Can you work these out from the model? Positions are in its coordinate system, mm. Face numbers are marked on the shaded views. A direction names the side the tool comes from. Give positions to 0.01 mm unless a question says otherwise; leave off trailing zeros. Order: outer loops, then holes, each group sorted by start corner. A loop starts at its lowest first (then second) coordinate and runs counter-clockwise, first axis right, second up. Notation, with made-up numbers: (55, 4.25) - (92, 4.25) arc R13 ccw to (92, 17.25) - close; hole circle Ø7 at (33, -28.75). An arc over 180 degrees is marked (long way). Use one line per item in the form item = value. Start each with the question number.
1) Suppose I cut it at B-B, the plane z = 4.5. Write out the boundary of the cut face in (x, y).
2) Which directions (+Z, -Z, +X, -X, +Y, -Y) give clear straight access to the entire face, cutting with the end or side of a thin tool? Please do the marked faces 3, 4 and 5.
3) Suppose I cut it at C-C, the plane z = -83.5. State how many separate pieces and enclosed holes the cut face has, and give its area (3 significant figures).
4) Please list where these lines run through material, in increasing order: probe 1 along X at (y, z) = (9.65, -70); probe 2 along X at (y, z) = (21, -66); probe 3 along X at (y, z) = (7, -24).
5) For pin 1 (0.6 mm diameter, centred on x = 0, y = 19.5, fed in from -Z); pin 2 (1.1 mm diameter, centred on x = -38, y = 20.5, fed in from +Z); pin 3 (3.5 mm diameter, centred on x = -39, z = -70.5, fed in from -Y), each with a flat end and sliding along its axis, tell me the tip position at first contact or that it passes through.
6) Suppose I cut it at A-A, the plane x = 21. Write out the boundary of the cut face in (y, z).
7) We'd pull the mould along X, two halves only. Please class the marked faces 1 and 2: released by +X, released by -X, zero draft, split by the parting line, or undercut.
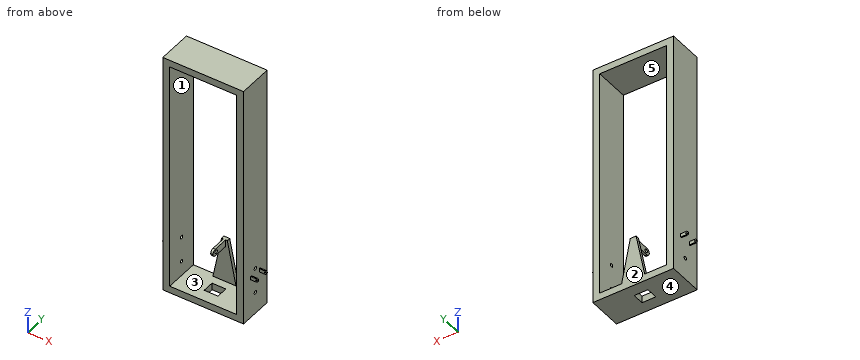
```python
from build123d import *

# Parameters (mm, degrees)
SKETCH1_W            = 70
SKETCH1_H            = 212
SKETCH1_W_2          = 58
SKETCH1_H_2          = 200
BOSS_EXTRUDE1_DEPTH  = 30
SKETCH10_W           = 2
SKETCH10_H           = 6
BOSS_EXTRUDE3_DEPTH  = 16
FILLET2_R            = 3
SKETCH2_R            = 1.5
CUT_EXTRUDE1_DEPTH   = 131.52202895
CUT_EXTRUDE2_REACH   = 218.954
SKETCH3_W            = 12
SKETCH3_H            = 10
SKETCH11_W           = 3
SKETCH11_H           = 1
BOSS_EXTRUDE4_DEPTH  = 6.3
FILLET3_R            = 1.5
SKETCH12_R           = 0.5
CUT_EXTRUDE3_DEPTH   = 116.683577146
FILLET3_OF_MIRROR1_R = 1.5


with BuildPart() as part:
    # Sketch1 → Boss-Extrude1 (new body)
    with BuildSketch(Plane(origin=(0, 0, 0), x_dir=(1, 0, 0), z_dir=(0, 1, 0))):
        Rectangle(SKETCH1_W, SKETCH1_H)
        Rectangle(SKETCH1_W_2, SKETCH1_H_2, mode=Mode.SUBTRACT)
    extrude(amount=BOSS_EXTRUDE1_DEPTH)

    # Sketch7 → Loft3 section 0
    with BuildSketch(Plane.XY.offset(-100)):
        with BuildLine():
            Line((-10, 30), (10, 30))
            Line((10, 30), (10, 27))
            Line((10, 27), (-10, 27))
            Line((-10, 27), (-10, 30))
        make_face()
    # Sketch8 → Loft3 section 1
    with BuildSketch(Plane.XY.offset(-62)):
        with BuildLine():
            Line((-2.5, 30), (2.5, 30))
            Line((2.5, 30), (2.5, 27))
            Line((2.5, 27), (-2.5, 27))
            Line((-2.5, 27), (-2.5, 30))
        make_face()
    loft()

    # Sketch10 → Boss-Extrude3 (add)
    with BuildSketch(Plane.XZ.offset(-27)):
        with Locations((0, -65)):
            Rectangle(SKETCH10_W, SKETCH10_H)
    extrude(amount=BOSS_EXTRUDE3_DEPTH)

    # Fillet2
    fillet2_edges = [part.edges().sort_by_distance(p)[0] for p in [
        (0, 11, -68),
        (0, 11, -62),
    ]]
    fillet(fillet2_edges, radius=FILLET2_R - 0.0001)  # a hair under: the kernel refuses the full size

    # Sketch2 → Cut-Extrude1 (cut, through all)
    with BuildSketch(Plane(origin=(35, 0, 0), x_dir=(0, 0, -1), z_dir=(1, 0, 0))):
        with Locations(Location((65, 15, 0), (0, 0, 270))):
            Circle(SKETCH2_R)
        with Locations((87, 15)):
            Circle(SKETCH2_R)
    extrude(amount=-CUT_EXTRUDE1_DEPTH, mode=Mode.SUBTRACT)

    # Sketch3 → Cut-Extrude2 (cut, up to next)
    with BuildSketch(Plane(origin=(0, 0, -106), x_dir=(-1, 0, 0), z_dir=(0, 0, -1)), mode=Mode.PRIVATE) as cut_extrude2_sk1:
        with Locations((0, 15)):
            Rectangle(SKETCH3_W, SKETCH3_H)
    cut_extrude2_tool1 = extrude(cut_extrude2_sk1.sketch, amount=-CUT_EXTRUDE2_REACH, mode=Mode.PRIVATE) & part.part
    add(cut_extrude2_tool1.solids().sort_by_distance((0, 15, -106))[0], mode=Mode.SUBTRACT)

    # Sketch11 → Boss-Extrude4 (add)
    with BuildSketch(Plane(origin=(35, 0, 0), x_dir=(0, 0, -1), z_dir=(1, 0, 0))):
        with Locations((70, 20.5)):
            Rectangle(SKETCH11_W, SKETCH11_H)
        with Locations((70, 9.5)):
            Rectangle(SKETCH11_W, SKETCH11_H)
    boss_extrude4 = extrude(amount=BOSS_EXTRUDE4_DEPTH)

    # Fillet3
    fillet3_edges = [part.edges().sort_by_distance(p)[0] for p in [
        (41.3, 9.5, -68.5),
        (41.3, 9.5, -71.5),
        (41.3, 20.5, -68.5),
        (41.3, 20.5, -71.5),
    ]]
    fillet(fillet3_edges, radius=FILLET3_R - 0.0001)  # a hair under: the kernel refuses the full size

    # Sketch12 → Cut-Extrude3 (cut, through all)
    with BuildSketch(Plane(origin=(0, 21, 0), x_dir=(1, 0, 0), z_dir=(0, 1, 0))):
        with Locations(Location((39.8, 70, 0), (0, 0, 270))):
            Circle(SKETCH12_R)
    cut_extrude3 = extrude(amount=-CUT_EXTRUDE3_DEPTH, mode=Mode.SUBTRACT)

    # Mirror1: Boss-Extrude4, Cut-Extrude3 across plane
    add(boss_extrude4.mirror(Plane(origin=(0, 0, 0), x_dir=(0, 0, 1), z_dir=(1, 0, 0))))
    add(cut_extrude3.mirror(Plane(origin=(0, 0, 0), x_dir=(0, 0, 1), z_dir=(1, 0, 0))), mode=Mode.SUBTRACT)

    # Fillet3 of Mirror1
    fillet3_of_mirror1_edges = [part.edges().sort_by_distance(p)[0] for p in [
        (-41.3, 9.5, -68.5),
        (-41.3, 9.5, -71.5),
        (-41.3, 20.5, -68.5),
        (-41.3, 20.5, -71.5),
    ]]
    fillet(fillet3_of_mirror1_edges, radius=FILLET3_OF_MIRROR1_R - 0.0001)  # a hair under: the kernel refuses the full size


solid = part.part
```
Result sheet:
q1.outline = (-35, 0) - (-29, 0) - (-29, 30) - (-35, 30) - close; (29, 0) - (35, 0) - (35, 30) - (29, 30) - close
q2.face_3 = -Y
q2.face_4 = -Z, +X, -X, +Y, -Y
q2.face_5 = +Y, -Y
q3.separate_pieces = 3
q3.enclosed_holes = 0
q3.area = 400 mm²
q4.probe_1 = -41.3 to -40.3, -39.3 to -29, 29 to 39.3, 40.3 to 41.3
q4.probe_2 = -35 to -29, -1 to 1, 29 to 35
q4.probe_3 = -35 to -29, 29 to 35
q5.pin_1 = -68
q5.pin_2 = -68.5
q5.pin_3 = 9
q6.outline = (0, -106) - (30, -106) - (30, -100) - (0, -100) - close; (0, 100) - (30, 100) - (30, 106) - (0, 106) - close
q7.face_1 = undercut
q7.face_2 = zero draft
